Could you check a few things on this model? Use its own coordinates, in mm. Face numbers are marked on the shaded views. A direction names the side the tool comes from. Give positions to 0.01 mm unless a question says otherwise; leave off trailing zeros. Loops run counter-clockwise (first coordinate to the right, second up) from the corner with the lowest first, then second, coordinate; pieces in that order, holes last.
1. For P1, Ø4, axis at x = 3, z = -1, coming from the -Y side; P2, Ø1.2, axis at x = 5.5, y = 5.5, coming from the -Z side; P3, Ø4, axis at x = 6, z = 0, coming from the +Y side; P4, Ø0.5, axis at x = 0, y = 5.5, coming from the +Z side, each with a flat end and sliding along its axis, tell me the tip position at first contact or that it passes through.
2. Imagine slicing it at A-A (z = -8). List the corners of the cut face in (x, y) for me.
3. Imagine slicing it at B-B (y = 1). List the corners of the cut face in (x, z) for me.
4. Imagine slicing it at C-C (x = 0.5). List the corners of the cut face in (y, z) for me.
5. I need wall thicknesses on line 1 along X through (y, z) = (2.05, 0); line 2 along X through (y, z) = (3.9, -16); line 3 along Y through (x, z) = (8.5, 3). Which ranges of each line are inside material? Lowest first, please.
6. For the marked faces 1, 2 and 3, which set-ups out of +Z, -Z, +X, -X, +Y, -Y let a thin tool reach every point of the face, with its end or its side?
7. Imagine slicing it at D-D (x = 7.25). List the corners of the cut face in (y, z) for me.
Autodesk Inventor part; units mm, degrees
ref_plane "YZ Plane" through (0, 0, 0) normal (1, 0, 0) x (0, 1, 0)
ref_plane "XZ Plane" through (0, 0, 0) normal (0, 1, 0) x (-1, 0, 0)
ref_plane "XY Plane" through (0, 0, 0) normal (0, 0, 1) x (1, 0, 0)
sketch "Sketch1" plane through (0, 0, 0) normal (0, 1, 0) x (-1, 0, 0)
  line L0 (4.2628, 17.0095) -> (-9.7372, 17.0095)
  line L1 (-9.7372, 17.0095) -> (-9.7372, -14.9905)
  line L2 (-9.7372, -14.9905) -> (4.2628, -14.9905)
  line L3 (4.2628, -14.9905) -> (4.2628, 17.0095)
  line L4 (4.7628, 17.5095) -> (-10.2372, 17.5095)
  line L5 (-10.2372, 17.5095) -> (-10.2372, -15.4905)
  line L6 (-10.2372, -15.4905) -> (4.7628, -15.4905)
  line L7 (4.7628, -15.4905) -> (4.7628, 17.5095)
  point P0 (0, 0)
  dimension "d0" = 14
  dimension "d1" = 32
  dimension "d2" = 0.5
extrude "Extrusion1" add sketch "Sketch1" along normal blind 2 contours L3 L2 L1 L0 | L7 L6 L5 L4
sketch "Sketch2" plane through (0, 2, 0) normal (0, 1, 0) x (1, 0, 0)
  line L0 (-4.7628, 15.4905) -> (-4.7628, -17.5095)
  line L1 (10.2372, -17.5095) -> (10.2372, 15.4905)
  line L2 (-3.2628, 15.4905) -> (-3.2628, -17.5095)
  line L3 (8.7372, -17.5095) -> (8.7372, 15.4905)
  line L4 (-3.2628, -17.5095) -> (-6.2628, -17.5095)
  line L5 (-6.2628, -17.5095) -> (-6.2628, 15.4905)
  line L6 (-6.2628, 15.4905) -> (-3.2628, 15.4905)
  line L7 (-3.2628, 15.4905) -> (-3.2628, -17.5095)
  line L8 (8.7372, -17.5095) -> (11.7372, -17.5095)
  line L9 (11.7372, -17.5095) -> (11.7372, 15.4905)
  line L10 (11.7372, 15.4905) -> (8.7372, 15.4905)
  line L11 (8.7372, 15.4905) -> (8.7372, -17.5095)
  point P0 (0, 0)
  dimension "d5" = 1.5
  dimension "d6" = 1.5
  dimension "d7" = 3
  dimension "d8" = 3
extrude "Extrusion2" add sketch "Sketch2" along normal blind 1
sketch "Sketch3" plane through (0, 3, 0) normal (0, 1, 0) x (1, 0, 0)
  line L0 (-6.2628, 15.4905) -> (-6.2628, -17.5095)
  line L1 (11.7372, -17.5095) -> (11.7372, 15.4905)
  line L2 (-6.2628, -17.5095) -> (-4.7628, -17.5095)
  line L3 (-3.2628, 15.4905) -> (-6.2628, 15.4905)
  line L4 (-6.2628, -17.5095) -> (-4.7628, -17.5095)
  line L5 (-4.7628, -17.5095) -> (-4.7628, 15.4905)
  line L6 (-4.7628, 15.4905) -> (-6.2628, 15.4905)
  line L7 (-6.2628, 15.4905) -> (-6.2628, -17.5095)
  line L8 (10.2372, -17.5095) -> (10.2372, 15.4905)
  line L9 (11.7372, -17.5095) -> (10.2372, -17.5095)
  line L10 (10.2372, -17.5095) -> (10.2372, 15.4905)
  line L11 (10.2372, 15.4905) -> (11.7372, 15.4905)
  line L12 (11.7372, 15.4905) -> (11.7372, -17.5095)
  point P0 (0, 0)
extrude "Extrusion3" add sketch "Sketch3" along normal blind 1.5
sketch "Sketch4" plane through (0, 4.5, 0) normal (0, 1, 0) x (1, 0, 0)
  line L0 (-4.7628, 15.4905) -> (-6.2628, 15.4905)
  line L1 (-6.2628, 15.4905) -> (-6.2628, -17.5095)
  line L2 (-6.2628, -17.5095) -> (-4.7628, -17.5095)
  line L3 (-4.7628, -17.5095) -> (-4.7628, 15.4905)
  line L4 (11.7372, -17.5095) -> (11.7372, 15.4905)
  line L5 (11.7372, 15.4905) -> (10.2372, 15.4905)
  line L6 (10.2372, 15.4905) -> (10.2372, -17.5095)
  line L7 (10.2372, -17.5095) -> (11.7372, -17.5095)
  line L8 (8.7372, 15.4905) -> (8.7372, -17.5095)
  line L9 (-3.2628, -17.5095) -> (-3.2628, 15.4905)
  line L10 (8.7372, 15.4905) -> (-3.2628, 15.4905)
  line L11 (-6.2628, -17.5095) -> (-3.2628, -17.5095)
  line L12 (-3.2628, -17.5095) -> (-3.2628, 15.4905)
  line L13 (-3.2628, 15.4905) -> (-6.2628, 15.4905)
  line L14 (-6.2628, 15.4905) -> (-6.2628, -17.5095)
  line L15 (11.7372, -17.5095) -> (8.7372, -17.5095)
  line L16 (8.7372, -17.5095) -> (8.7372, 15.4905)
  line L17 (8.7372, 15.4905) -> (11.7372, 15.4905)
  line L18 (11.7372, 15.4905) -> (11.7372, -17.5095)
  point P0 (0, 0)
extrude "Extrusion4" add sketch "Sketch4" along normal blind 1.5
chamfer "Chamfer1" distance 0.5 angle 45 4 edges at (-3.2628, 3, 1.0095) (8.7372, 3, 1.0095) (10.2372, 3, 1.0095) (-4.7628, 3, 1.0095)
chamfer "Chamfer2" distance 0.5 angle 45 4 edges at (-4.7628, 4.5, 1.0095) (10.2372, 4.5, 1.0095) (8.7372, 4.5, 1.0095) (-3.2628, 4.5, 1.0095)
sketch "Sketch5" plane through (0, 2, 0) normal (0, -1, 0) x (1, 0, 0)
  line L0 (-4.7628, -15.4905) -> (-4.7628, 17.5095)
  line L1 (-6.2628, 17.5095) -> (-4.7628, 17.5095)
  line L2 (-6.2628, -15.4905) -> (-6.2628, 17.5095)
  line L3 (-4.7628, -15.4905) -> (-6.2628, -15.4905)
  line L4 (10.2372, 17.5095) -> (10.2372, -15.4905)
  line L5 (11.7372, -15.4905) -> (10.2372, -15.4905)
  line L6 (11.7372, 17.5095) -> (11.7372, -15.4905)
  line L7 (10.2372, 17.5095) -> (11.7372, 17.5095)
  point P0 (0, 0)
extrude "Extrusion5" add sketch "Sketch5" along normal up to surface (2 mm away)
sketch "Sketch6" plane through (11.7372, 0, -15.4905) normal (0, 0, -1) x (-1, 0, 0)
  line L0 (0, 0) -> (0, 6)
  line L1 (18, 0) -> (0, 0)
  line L2 (0, 6) -> (3, 6)
  line L3 (15, 6) -> (18, 6)
  line L4 (18, 0) -> (18, 6)
  line L5 (16.5, 4) -> (16, 4.5)
  line L6 (15.5, 4.5) -> (16, 4.5)
  line L7 (16.5, 3.5) -> (16.5, 4)
  line L8 (16, 3) -> (16.5, 3.5)
  line L9 (15.5, 3) -> (16, 3)
  line L10 (2, 3) -> (2.5, 3)
  line L11 (1.5, 3.5) -> (2, 3)
  line L12 (1.5, 3.5) -> (1.5, 4)
  line L13 (2, 4.5) -> (1.5, 4)
  line L14 (2, 4.5) -> (2.5, 4.5)
  line L15 (2.5, 4.5) -> (15.5, 4.5)
  line L16 (3, 2.5) -> (2.5, 3)
  line L17 (15, 2.5) -> (15.5, 3)
  line L18 (2.5, 3) -> (15.5, 3)
  line L19 (3, 5) -> (3, 6)
  line L20 (15, 5) -> (15, 6)
  line L21 (3, 6) -> (15, 6)
  point P0 (11.7372, 0)
extrude "Extrusion6" add sketch "Sketch6" along normal blind 1.5
sketch "Sketch7" plane through (11.7372, 0, -16.9905) normal (0, 0, -1) x (-1, 0, 0)
  line L0 (0, 6) -> (0, 0)
  line L1 (0, 0) -> (18, 0)
  line L2 (18, 6) -> (18, 0)
  line L3 (0, 6) -> (18, 6)
  line L4 (18, 6) -> (18, 0)
  line L5 (18, 0) -> (0, 0)
  line L6 (0, 0) -> (0, 6)
  point P0 (11.7372, 0)
extrude "Extrusion7" add sketch "Sketch7" along normal blind 1.5
chamfer "Chamfer3" distance 0.5 angle 45 2 edges at (2.7372, 3, -15.4905) (2.7372, 4.5, -15.4905)
sketch "Sketch8" plane through (11.7372, 0, -18.4905) normal (0, 0, -1) x (-1, 0, 0)
  line L0 (0, 6) -> (0, 0)
  line L1 (0, 0) -> (18, 0)
  line L2 (18, 0) -> (18, 6)
  line L3 (18, 6) -> (0, 6)
  point P0 (11.7372, 0)
extrude "Extrusion8" add sketch "Sketch8" along normal blind 10
sketch "Sketch9" plane through (0, 6, 0) normal (0, 1, 0) x (1, 0, 0)
  line L0 (-6.2628, 28.4905) -> (11.7372, 28.4905)
  line L1 (-6.2628, -17.5095) -> (-6.2628, 28.4905)
  line L2 (11.7372, 28.4905) -> (-6.2628, 28.4905)
  line L3 (-6.2628, 28.4905) -> (-6.2628, 18.4905)
  line L4 (-6.2628, 18.4905) -> (11.7372, 18.4905)
  line L5 (11.7372, 18.4905) -> (11.7372, 28.4905)
  point P0 (0, 0)
  dimension "d32" = 10
extrude "Extrusion9" cut sketch "Sketch9" against normal blind 3
sketch "Sketch10" plane through (0, 3, 0) normal (0, 1, 0) x (1, 0, 0)
  line L0 (11.7372, 28.4905) -> (11.7372, 18.4905)
  line L1 (-6.2628, 18.4905) -> (-6.2628, 28.4905)
  line L2 (11.7372, 18.4905) -> (-6.2628, 18.4905)
  line L3 (11.7372, 28.4905) -> (-6.2628, 18.4905)
  circle A0 centre (2.7372, 23.4905) radius 1.5
  point P0 (0, 0)
  dimension "d35" = 3
extrude "Extrusion10" cut sketch "Sketch10" against normal blind 3 contours A0 L3 | L3 A0
fillet "Fillet1" radius 8 2 edges at (-6.2628, 1.5, -28.4905) (11.7372, 1.5, -28.4905)
chamfer "Chamfer4" distance 1.5 angle 45 1 edges at (2.7372, 3, -18.4905)
properties part number "RC_Snubber_3DPrint"
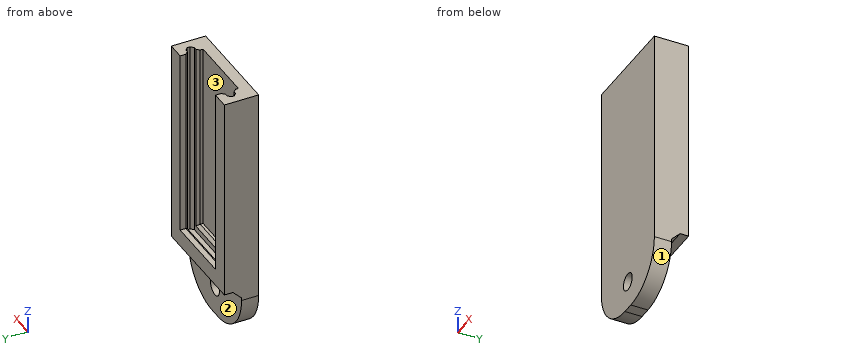
Derived:
1. P1: stops at y = 0
1. P2: stops at z = -18.49
1. P3: stops at y = 2
1. P4: stops at z = -15.49
2. outline: (-6.26, 0) - (11.74, 0) - (11.74, 6) - (8.74, 6) - (8.74, 5) - (9.24, 4.5) - (9.74, 4.5) - (10.24, 4) - (10.24, 3.5) - (9.74, 3) - (9.24, 3) - (8.74, 2.5) - (8.74, 2) - (-3.26, 2) - (-3.26, 2.5) - (-3.76, 3) - (-4.26, 3) - (-4.76, 3.5) - (-4.76, 4) - (-4.26, 4.5) - (-3.76, 4.5) - (-3.26, 5) - (-3.26, 6) - (-6.26, 6) - close
3. outline: (-6.26, -20.49) arc R8 ccw to (1.74, -28.49) - (3.74, -28.49) arc R8 ccw to (11.74, -20.49) - (11.74, 17.51) - (-6.26, 17.51) - close; hole circle Ø3 at (2.74, -23.49)
4. outline: (0, -28.39) - (3, -28.39) - (3, -19.99) - (4.5, -18.49) - (6, -18.49) - (6, -15.49) - (5, -15.49) - (4.5, -15.99) - (4.5, -16.99) - (3, -16.99) - (3, -15.99) - (2.5, -15.49) - (2, -15.49) - (2, 17.51) - (0, 17.51) - close
5. line 1: x = -6.26 to -3.26, 8.74 to 11.74
5. line 2: x = -6.26 to -4.76, 10.24 to 11.74
5. line 3: y = 0 to 2
6. face 1: -Z, +X, +Y, -Y
6. face 2: -Z, +X, -X, +Y
6. face 3: +Z, +Y
7. outline: (0, -27.68) - (3, -27.68) - (3, -19.99) - (4.5, -18.49) - (6, -18.49) - (6, -15.49) - (5, -15.49) - (4.5, -15.99) - (4.5, -16.99) - (3, -16.99) - (3, -15.99) - (2.5, -15.49) - (2, -15.49) - (2, 17.51) - (0, 17.51) - close
